```python
from build123d import *

# Parameters (mm, degrees)
CHAMFER1_SIZE = 0.2


with BuildPart() as part:
    # Sketch1 → Revolve1 (revolve)
    with BuildSketch(Plane(origin=(0, 0, 0), x_dir=(0, 0, -1), z_dir=(1, 0, 0)), mode=Mode.PRIVATE) as revolve1_sk:
        with BuildLine():
            Line((-1.80638465, 0), (2.358456395, 0))
            Line((2.358456395, 0), (4.154321235, 0))
            Line((4.154321235, 0), (4.154321235, 2))
            Line((4.154321235, 2), (2.754321235, 2))
            Line((2.754321235, 2), (2.754321235, 1.381443299))
            Line((2.754321235, 1.381443299), (2.154321235, 1.381443299))
            Line((2.154321235, 1.381443299), (2.154321235, 2))
            Line((2.154321235, 2), (-1.845678765, 2))
            Line((-1.845678765, 2), (-1.845678765, 2.410234036))
            ThreePointArc((-1.845678765, 2.410234036), (-2.687941743, 1.981004397), (-3.368605566, 1.325))
            Line((-3.368605566, 1.325), (-3.368605566, 0))
            Line((-3.368605566, 0), (-1.80638465, 0))
        make_face()
    revolve(revolve1_sk.sketch.rotate(Axis((0, 0, 1.80638465), (0, 0, -1)), 90), axis=Axis((0, 0, 1.80638465), (0, 0, -1)))

    # Chamfer1
    chamfer1_edges = [part.edges().sort_by_distance(p)[0] for p in [
        (-2, 0, -4.154321235),
    ]]
    chamfer(chamfer1_edges, length=CHAMFER1_SIZE)


solid = part.part
```
Can you work these out from the model? Positions are in its coordinate system, mm. Give positions to 0.01 mm unless a question says otherwise; leave off trailing zeros. Use a Markdown table: item, result. Add a question column.
Q1. I'm going to push flat-ended pins straight in: pin 1 (1.5 mm diameter, centred on y = -1.5, z = 0, fed in from -X); pin 2 (1 mm diameter, centred on y = -1, z = 1.5, fed in from +X). Where does each tip first touch, or does it pass through?
Q2. If we mould it in two halves opening along Z, with no side actions, what happens to faces 1 (the flat face through (0, 0, -4.154)), 2 (the cylindrical face through (1.32, -0.41, -2.45)), 3 (the cylindrical face through (0, 2, -3)), 4 (the flat face through (0, 0, 3.369))? For each: released by +Z, released by -Z, zero draft, split by the parting line, or undercut.
Q3. Please list where these lines run through material, in increasing order: line 1 along Y through (x, z) = (0.1, -1); line 2 along Z through (x, y) = (-1.4, -1.05); line 3 along X through (y, z) = (1.5, -3.25).
Answers follow:
| question | item | result |
|---|---|---|
| 1 | pin 1 | stops at x = -1.85 |
| 1 | pin 2 | stops at x = 2.32 |
| 2 | face 1 | released by -Z |
| 2 | face 2 | undercut |
| 2 | face 3 | zero draft |
| 2 | face 4 | released by +Z |
| 3 | line 1 | y = -2 to 2 |
| 3 | line 2 | z = -4.15 to -2.75, -2.15 to 2.98 |
| 3 | line 3 | x = -1.32 to 1.32 |
